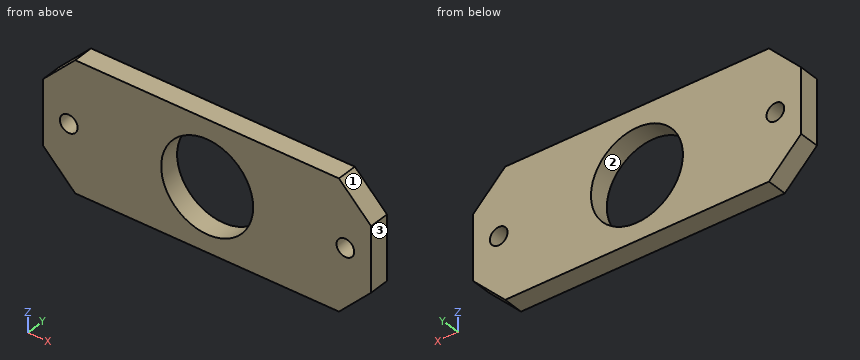
from build123d import *

# Parameters (mm, degrees)
SKETCH1_W           = 82
SKETCH1_H           = 70
BOSS_EXTRUDE1_DEPTH = 6.35
SKETCH4_R           = 14.295
CUT_EXTRUDE3_DEPTH  = 7.35
SKETCH7_W           = 70
SKETCH7_H           = 6.35
BOSS_EXTRUDE2_DEPTH = 10
SKETCH8_W           = 70
SKETCH8_H           = 6.35
BOSS_EXTRUDE3_DEPTH = 10
SKETCH6_R           = 2.75
CUT_EXTRUDE4_DEPTH  = 10
CHAMFER1_SIZE       = 25
SKETCH9_OUTSIDE_W   = 128.774
SKETCH9_OUTSIDE_H   = 96.774
SKETCH9_OUTSIDE_W_2 = 112.086128576
SKETCH9_OUTSIDE_H_2 = 40
CUT_EXTRUDE6_DEPTH  = 6.35


with BuildPart() as part:
    # Sketch1 → Boss-Extrude1 (new body)
    with BuildSketch(Plane(origin=(0, 0, 0), x_dir=(1, 0, 0), z_dir=(0, 1, 0))):
        with Locations((40.204600864, 28.763107794)):
            Rectangle(SKETCH1_W, SKETCH1_H)
    extrude(amount=BOSS_EXTRUDE1_DEPTH)

    # Sketch4 → Cut-Extrude3 (cut, through all)
    with BuildSketch(Plane(origin=(0, 6.35, 0), x_dir=(1, 0, 0), z_dir=(0, 1, 0))):
        with Locations((40.245025705, 29.040694999)):
            Circle(SKETCH4_R)
    extrude(amount=-CUT_EXTRUDE3_DEPTH, mode=Mode.SUBTRACT)

    # Sketch7 → Boss-Extrude2 (add)
    with BuildSketch(Plane.ZY.offset(0.795399136)):
        with Locations((-28.763107794, 3.175)):
            Rectangle(SKETCH7_W, SKETCH7_H)
    extrude(amount=BOSS_EXTRUDE2_DEPTH)

    # Sketch8 → Boss-Extrude3 (add)
    with BuildSketch(Plane(origin=(81.204600864, 0, 0), x_dir=(0, 0, -1), z_dir=(1, 0, 0))):
        with Locations((28.763107794, 3.175)):
            Rectangle(SKETCH8_W, SKETCH8_H)
    extrude(amount=BOSS_EXTRUDE3_DEPTH)

    # Sketch6 → Cut-Extrude4 (cut)
    with BuildSketch(Plane.XZ):
        with Locations((-2.795399136, -28.763107793)):
            Circle(SKETCH6_R)
        with Locations((83.204600864, -28.763107784)):
            Circle(SKETCH6_R)
    extrude(amount=-CUT_EXTRUDE4_DEPTH, mode=Mode.SUBTRACT)

    # Chamfer1
    chamfer1_edges = [part.edges().sort_by_distance(p)[0] for p in [
        (-10.795399136, 3.175, 6.236892206),
        (-10.795399136, 3.175, -63.763107794),
        (91.204600864, 3.175, 6.236892206),
        (91.204600864, 3.175, -63.763107794),
    ]]
    chamfer(chamfer1_edges, length=CHAMFER1_SIZE)

    # Sketch9 outside → Cut-Extrude6 (cut)
    with BuildSketch(Plane.XZ):
        with Locations((40.205, -28.763)):
            Rectangle(SKETCH9_OUTSIDE_W, SKETCH9_OUTSIDE_H)
        with Locations((41.847145894, -28.763107784)):
            Rectangle(SKETCH9_OUTSIDE_W_2, SKETCH9_OUTSIDE_H_2, mode=Mode.SUBTRACT)
    extrude(amount=-CUT_EXTRUDE6_DEPTH, mode=Mode.SUBTRACT)


solid = part.part
CAD build for the part. Positions are in the model's coordinates, mm. Face numbers are marked on the shaded views. Coordinates: 2 decimals unless noted, no trailing zeros. Write each loop counter-clockwise with the first axis right and the second up, starting at its lowest first coordinate (ties: lowest second). Pieces come first, ordered by that corner, then holes. Notation, with made-up numbers: M -30.5,71.25 L -24.5,71.25 A13 cw -24.5,87.25 Z; hole C 7.5,1 d9. An arc over 180 degrees is marked long. Answer as a JSON object with one key per item and string values. Group by question number.
1) Saw through at D-D (z = -45). Write the cut outline in (x, y), plus the area to 3 significant figures.
2) Mould opens along Z. For the marked faces 1, 2 and 3 say: +Z half, -Z half, draft (parallel to the pull), parting line (faces both ways), or undercut.
3) Wall check: line 1 (X direction, y = 0.75, z = -20); line 2 (Z direction, x = -3.5, y = 1.25); line 3 (X direction, y = 0.5, z = -27.5). Give the ranges that are in metal, low to high. Write a range as from..to.
4) Pin check, flat tips, straight feed: pin 1 Ø4.5 at (x, z) = (-2.8, -28.76) entering from +Y; pin 2 Ø9 at (x, z) = (83.2, -28.76) entering from -Y. Stop position of each tip, or through.
5) Saw through at A-A (z = -32.5). Write the cut outline in (x, y).
6) Saw through at C-C (y = 2.25). Write the cut outline in (x, z) (3 decimals).
7) Saw through at B-B (x = 28). Write the cut outline in (y, z).
Values follow:
{
 "1": {"outline": "M -4.56,0 L 84.97,0 L 84.97,6.35 L -4.56,6.35 Z", "area": "568 mm2"},
 "2": {"face 1": "+Z half", "face 2": "undercut", "face 3": "draft"},
 "3": {"line 1": "x = -10.8..29.17, 51.32..91.2", "line 2": "z = -46.06..-31.42, -26.1..-11.47", "line 3": "x = -10.8..-5.24, -0.35..26.03, 54.46..80.76, 85.65..91.2"},
 "4": {"pin 1": "passes through", "pin 2": "stops at y = 0"},
 "5": {"outline": "M -10.8,0 L 26.37,0 L 26.37,6.35 L -10.8,6.35 Z; M 54.12,0 L 91.2,0 L 91.2,6.35 L 54.12,6.35 Z"},
 "6": {"outline": "M -10.795,-38.763 L -0.795,-48.763 L 81.205,-48.763 L 91.205,-38.763 L 91.205,-18.763 L 81.205,-8.763 L -0.795,-8.763 L -10.795,-18.763 Z; hole C -2.795,-28.763 d5.5; hole C 40.245,-29.041 d28.59; hole C 83.205,-28.763 d5.5"},
 "7": {"outline": "M 0,-48.76 L 6.35,-48.76 L 6.35,-36.42 L 0,-36.42 Z; M 0,-21.66 L 6.35,-21.66 L 6.35,-8.76 L 0,-8.76 Z"}
}
